from build123d import *

# Parameters (mm, degrees)
SKICA1_W                 = 50
SKICA1_H                 = 10
P_IDAT_VYSUNUT_M1_DEPTH  = 8
SKICA2_R                 = 1.65
ODEBRAT_VYSUNUT_M1_DEPTH = 52.613951602
ZAOBLIT2_R               = 5
SKICA3_R                 = 3
ODEBRAT_VYSUNUT_M2_DEPTH = 2.5
ODEBRAT_VYSUNUT_M3_DEPTH = 2.5


with BuildPart() as part:
    # Skica1 → Přidat vysunutím1 (new body)
    with BuildSketch(Plane.XY):
        with Locations((25, 5)):
            Rectangle(SKICA1_W, SKICA1_H)
    extrude(amount=P_IDAT_VYSUNUT_M1_DEPTH)

    # Skica2 → Odebrat vysunutím1 (cut, through all)
    with BuildSketch(Plane.XY.offset(8)):
        with Locations((5, 5)):
            Circle(SKICA2_R)
        with Locations((45, 5)):
            Circle(SKICA2_R)
    extrude(amount=-ODEBRAT_VYSUNUT_M1_DEPTH, mode=Mode.SUBTRACT)

    # Zaoblit2
    zaoblit2_edges = [part.edges().sort_by_distance(p)[0] for p in [
        (50, 0, 4),
        (50, 10, 4),
        (0, 0, 4),
        (0, 10, 4),
    ]]
    fillet(zaoblit2_edges, radius=ZAOBLIT2_R - 0.0001)  # a hair under: the kernel refuses the full size

    # Skica3 → Odebrat vysunutím2 (cut)
    with BuildSketch(Plane.XY.offset(8)):
        with Locations((45, 5)):
            Circle(SKICA3_R)
    extrude(amount=-ODEBRAT_VYSUNUT_M2_DEPTH, mode=Mode.SUBTRACT)

    # Skica4 → Odebrat vysunutím3 (cut)
    with BuildSketch(Plane(origin=(0, 0, 0), x_dir=(-1, 0, 0), z_dir=(0, 0, -1))):
        Polygon((-6.58771324, 7.75), (-8.175426481, 5), (-6.58771324, 2.25), (-3.41228676, 2.25), (-1.824573519, 5), (-3.41228676, 7.75), align=None)
    extrude(amount=-ODEBRAT_VYSUNUT_M3_DEPTH, mode=Mode.SUBTRACT)


solid = part.part
Read the model definition and answer for the solid it produces. Units are mm, in the model's axes. A direction names the side the tool comes from. Coordinates: 2 decimals unless noted, no trailing zeros. Return JSON: item names as keys, results as strings.
(1) Consider line 1 along Y through (x, z) = (5, 5.3); line 2 along X through (y, z) = (6, 3.75); line 3 along X through (y, z) = (4.75, 2.75). Determine where each line is inside the solid, lowest interval first. Write a range as from..to.
Answers below:
{"line 1": "0..3.35, 6.65..10", "line 2": "0.1..3.69, 6.31..43.69, 46.31..49.9", "line 3": "0.01..3.37, 6.63..43.37, 46.63..49.99"}
(2) The part is cut by section A-A on z = 0.5. State how many separate pieces and enclosed holes the cut face has, then the cut area to 3 significant figures.
Answers below:
{"separate pieces": "1", "enclosed holes": "2", "area": "444 mm^2"}
(3) Which of the six approach directions +Z, -Z, +X, -X, +Y, -Y give full straight-line access (tool end or side, diameter ignored) to faces 5 (the flat face through (5, 7.75, 1)), 6 (the flat face through (46.3, 3.7, 5.5)), 7 (the flat face through (25, 5, 8))?
Answers below:
{"face 5": "-Z", "face 6": "+Z", "face 7": "+Z, +X, -X, +Y, -Y"}
(4) For a pull along X with two mould halves and no side action, classify faces 1 (the flat face through (7.39, 3.64, 1.23)), 2 (the cylindrical face through (48, 9, 4)), 3 (the cylindrical face through (1, 2, 4)), 4 (the flat face through (25, 5, 0)) as pulls with the +X half, pulls with the -X half, needs draft (parallel to the pull), parting line crosses it, or undercut.
Answers below:
{"face 1": "undercut", "face 2": "pulls with the +X half", "face 3": "pulls with the -X half", "face 4": "needs draft"}
(5) Each of these flat-tipped pins is pushed along its axis until it touches: P1, Ø1.6, axis at x = 6.5, y = 6, coming from the -Z side; P2, Ø3, axis at x = 5, y = 5, coming from the +Z side; P3, Ø3, axis at y = 7, z = 4.5, coming from the -X side. Where does it stop, or does it pass through?
Answers below:
{"P1": "z = 2.5", "P2": "through", "P3": "x = 0.03"}
